Autodesk Inventor part; units mm, degrees
ref_plane "工作平面1" through (12, 0, 0) normal (1, 0, 0) x (0, 1, 0)
ref_plane "XZ Plane" through (0, 0, 0) normal (0, 1, 0) x (-1, 0, 0)
ref_plane "XY Plane" through (0, 0, 0) normal (0, 0, 1) x (1, 0, 0)
sketch "草图1" plane through (0, 0, 0) normal (0, 1, 0) x (-1, 0, 0)
  circle A0 centre (0, 0) radius 10.1
  circle A1 centre (0, 0) radius 15
  dimension "d0" = 20.2
  dimension "d1" = 30
extrude "拉伸1" add sketch "草图1" along normal blind 6
ref_plane "工作平面1" through (12, 0, 0) normal (1, 0, 0) x (0, 1, 0)
sketch "草图2" plane through (12, 0, 0) normal (1, 0, 0) x (0, 1, 0)
  line L0 (6, -15) -> (6, 15) construction
  line L1 (6, -6) -> (0, -6)
  line L2 (0, -6) -> (0, 6) construction
  line L3 (0, -15) -> (0, 15) construction
  line L4 (6, 6) -> (6, -6) construction
  line L5 (0, 6) -> (6, 6)
  line L6 (6, 0) -> (0, 0)
  line L7 (6, 6) -> (6, 4)
  line L8 (6, 4) -> (4.75, 4)
  line L9 (4.75, 4) -> (4.75, -4)
  line L10 (4.75, -4) -> (6, -4)
  line L11 (6, -4) -> (6, -6)
  line L12 (0, -6) -> (0, -4)
  line L13 (1.25, -4) -> (0, -4)
  line L14 (1.25, -4) -> (1.25, 4)
  line L15 (1.25, 4) -> (0, 4)
  line L16 (0, 6) -> (0, 4)
  line L17 (3, 6) -> (3, -6)
  dimension "d5" = 12
  dimension "d6" = 2
  dimension "d7" = 3.5
extrude "拉伸2" add sketch "草图2" along normal blind 35
sketch "草图3" plane through (0, 0, 0) normal (0, 1, 0) x (-1, 0, 0)
  line L0 (-47, 4) -> (-47, -4)
  circle A0 centre (-47, 0) radius 6
  circle A1 centre (-47, 0) radius 3.6
  point P0 (0, 0)
  point P1 (-47, -6)
  dimension "d10" = 7.2
extrude "拉伸3" cut sketch "草图3" along normal mid plane 35 contours A1 L0 | L0 A1
extrude "拉伸4" add sketch "草图3" along normal blind 6
properties part number "偏心轮外连接件"
Geometry: final body of the model. Coordinates: model frame, mm. A direction names the side the tool comes from. Give positions to 0.01 mm unless a question says otherwise; leave off trailing zeros. Loops run counter-clockwise (first coordinate to the right, second up) from the corner with the lowest first, then second, coordinate; pieces in that order, holes last. Notation, with made-up numbers: (-19, 35.25) -> (29, 35.25) arc R19 cw to (29, 42.25) -> close; hole circle Ø11 at (50.5, 46). An arc over 180 degrees is marked (long way). Return JSON: item names as keys, results as strings.
Item 1: Mould query, pull axis X, two halves, no side actions, for faces 4 (the cylindrical face through (53, 3, 0)), 5 (the cylindrical face through (-9.634, 2.958, -3.034)), 6 (the flat face through (12, 6, 1)). Classes: released by +X, released by -X, zero draft, split by the parting line, or undercut.
Filled in:
{"face 4": "released by +X", "face 5": "undercut", "face 6": "zero draft"}
Item 2: Line query: line 1 (Z direction, x = 0, y = 4.35); line 2 (Z direction, x = 47, y = 2.8); line 3 (Z direction, x = 16, y = 4.65). Output: solid intervals per line, ascending.
Filled in:
{"line 1": "-15 to -10.1, 10.1 to 15", "line 2": "-6 to -3.6, 3.6 to 6", "line 3": "-6 to 6"}
Item 3: Access query for faces 1 (the flat face through (28, 5, 4)), 2 (the flat face through (30, 3, 6)), 3 (the flat face through (30, 3, -6)). Directions: +Z, -Z, +X, -X, +Y, -Y. A direction counts if a zero-diameter tool reaches every point of the face in a straight line with its end or side. Return the directions, or none.
Filled in:
{"face 1": "+Y", "face 2": "+Z, +X, +Y, -Y", "face 3": "-Z, +X, +Y, -Y"}
Item 4: Section C-C, the plane x = 26. Output: boundary loops of the cut face in (y, z), plus the area to 3 significant figures.
Filled in:
{"outline": "(0, -6) -> (6, -6) -> (6, -4) -> (4.75, -4) -> (4.75, 4) -> (6, 4) -> (6, 6) -> (0, 6) -> (0, 4) -> (1.25, 4) -> (1.25, -4) -> (0, -4) -> close", "area": "52.0 mm^2"}
Item 5: Section B-B, the plane z = -2.5. Output: boundary loops of the cut face in (x, y).
Filled in:
{"outline": "(-14.79, 0) -> (-9.79, 0) -> (-9.79, 6) -> (-14.79, 6) -> close; (9.79, 0) -> (14.79, 0) -> (14.79, 1.25) -> (41.55, 1.25) -> (41.55, 0) -> (44.41, 0) -> (44.41, 6) -> (41.55, 6) -> (41.55, 4.75) -> (14.79, 4.75) -> (14.79, 6) -> (9.79, 6) -> close; (49.59, 0) -> (52.45, 0) -> (52.45, 6) -> (49.59, 6) -> close"}
Item 6: Section A-A, the plane x = 0. Output: boundary loops of the cut face in (y, z), plus the area to 3 significant figures.
Filled in:
{"outline": "(0, -15) -> (6, -15) -> (6, -10.1) -> (0, -10.1) -> close; (0, 10.1) -> (6, 10.1) -> (6, 15) -> (0, 15) -> close", "area": "58.8 mm^2"}
Item 7: Section D-D, the plane z = -12. Output: boundary loops of the cut face in (x, y), plus the area to 3 significant figures.
Filled in:
{"outline": "(-9, 0) -> (9, 0) -> (9, 6) -> (-9, 6) -> close", "area": "108 mm^2"}
Item 8: Pin query (flat end, axial travel): P1, Ø2, axis at x = 16.5, y = 4, coming from the +Z side; P2, Ø2.5, axis at x = 26, z = -1, coming from the +Y side; P3, Ø1.8, axis at x = 35, y = 3.5, coming from the -Z side; P4, Ø18, axis at x = 0, z = 0, coming from the +Y side. Return the tip coordinate at first contact, or that it passes through.
Filled in:
{"P1": "z = 6", "P2": "y = 4.75", "P3": "z = -6", "P4": "through"}
